from build123d import *

# Parameters (mm, degrees)
BOSS_EXTRUDE1_DEPTH = 406.4
SKETCH2_R           = 2.38125
CUT_EXTRUDE1_DEPTH  = 411.349558304
CHAMFER1_SIZE       = 50.8
CHAMFER2_SIZE       = 50.8


with BuildPart() as part:
    # Sketch1 → Boss-Extrude1 (new body)
    with BuildSketch(Plane.XY):
        Polygon((0, 25.4), (0, 0), (50.8, 0), (50.8, 3.175), (3.175, 3.175), (3.175, 25.4), align=None)
    extrude(amount=BOSS_EXTRUDE1_DEPTH)

    # Sketch2 → Cut-Extrude1 (cut, through all)
    with BuildSketch(Plane.ZY):
        with Locations((381, 12.7)):
            Circle(SKETCH2_R)
        with Locations((330.2, 12.7)):
            Circle(SKETCH2_R)
        with Locations((279.4, 12.7)):
            Circle(SKETCH2_R)
        with Locations((228.6, 12.7)):
            Circle(SKETCH2_R)
        with Locations((177.8, 12.7)):
            Circle(SKETCH2_R)
        with Locations((127, 12.7)):
            Circle(SKETCH2_R)
        with Locations((76.2, 12.7)):
            Circle(SKETCH2_R)
        with Locations((25.4, 12.7)):
            Circle(SKETCH2_R)
        with Locations((-25.4, 12.7)):
            Circle(SKETCH2_R)
        with Locations((-76.2, 12.7)):
            Circle(SKETCH2_R)
    extrude(amount=-CUT_EXTRUDE1_DEPTH, mode=Mode.SUBTRACT)

    # Chamfer1
    chamfer1_edges = [part.edges().sort_by_distance(p)[0] for p in [
        (50.8, 1.5875, 406.4),
    ]]
    chamfer(chamfer1_edges, length=CHAMFER1_SIZE - 0.0001)  # a hair under: the kernel refuses the full size

    # Chamfer2
    chamfer2_edges = [part.edges().sort_by_distance(p)[0] for p in [
        (50.8, 1.5875, 0),
    ]]
    chamfer(chamfer2_edges, length=CHAMFER2_SIZE - 0.0001)  # a hair under: the kernel refuses the full size


solid = part.part
Source: CAD feature listing. Evaluate the final solid. Frame: model axes, mm. A direction names the side the tool comes from. Coordinates: 2 decimals unless noted, no trailing zeros. Loops run counter-clockwise (first coordinate to the right, second up) from the corner with the lowest first, then second, coordinate; pieces in that order, holes last. Notation, with made-up numbers: M 46,0.25 L 102,0.25 A19 ccw 102,9.25 Z; hole C 51,-12.75 d5. An arc over 180 degrees is marked long. Answer in a Markdown table with one row per item.
Q1. First-contact query: pin 1 (1 mm diameter, centred on y = 23, z = 331, fed in from +X) (3 decimals); pin 2 (3 mm diameter, centred on y = 12.7, z = 127, fed in from +X); pin 3 (10 mm diameter, centred on x = 10.5, y = 4.5, fed in from -Z). Flat tips, straight axial feed; report the tip coordinate or a pass-through.
Answers below:
| item | result |
|---|---|
| pin 1 | stops at x = 3.175 |
| pin 2 | passes through |
| pin 3 | stops at z = 5.68 |
Q2. Section A-A on z = 139. Return the cut outline in (x, y) (3 decimals).
Answers below:
| item | result |
|---|---|
| outline | M 0,0 L 50.8,0 L 50.8,3.175 L 3.175,3.175 L 3.175,25.4 L 0,25.4 Z |
Q3. Set-up query: faces 1 (the flat face through (18, 2, 18)), 2 (the flat face through (3.175, 14, 200)). Return all of +Z, -Z, +X, -X, +Y, -Y with unobstructed straight access to the full face (end or side cutting, diameter ignored); none if empty.
Answers below:
| item | result |
|---|---|
| face 1 | -Z, +X, +Y, -Y |
| face 2 | +Z, -Z, +X, +Y |
Q4. Ray query, probe 1 along Y at (x, z) = (0.7, 330.2); probe 2 along Y at (x, z) = (36, 313.5) (3 decimals). Return the intervals inside material, ascending. Write a range as from..to.
Answers below:
| item | result |
|---|---|
| probe 1 | y = 0..10.32, 15.08..25.4 |
| probe 2 | y = 0..3.175 |
Q5. Section B-B on x = 29.5. Return the cut outline in (y, z) (3 decimals).
Answers below:
| item | result |
|---|---|
| outline | M 0,29.5 L 3.175,29.5 L 3.175,376.9 L 0,376.9 Z |
